```python
from build123d import *

# Parameters (mm, degrees)
F0_W       = 34
F0_H       = 18
F1_DEPTH   = 80
F2_SIZE2   = 7
F2_SIZE    = 17
F2_2_SIZE2 = 7
F2_2_SIZE  = 17
F3_T       = -1.2
F5_DEPTH   = 18.001
F6_R       = 1.2
F7_R       = 2.4


with BuildPart() as f1:
    # F0 (on Top) → F1 (new body)
    with BuildSketch(Plane.XY):
        Rectangle(F0_W, F0_H)
    extrude(amount=F1_DEPTH)

    # F2
    f2_edges = [f1.edges().sort_by_distance(p)[0] for p in [
        (-17, 0, 80),
    ]]
    f2_side = f1.faces().sort_by_distance((-17, 0, 40))[0]
    chamfer(f2_edges, length=F2_SIZE, length2=F2_SIZE2, reference=f2_side)

    # F2#2
    f2_2_edges = [f1.edges().sort_by_distance(p)[0] for p in [
        (17, 0, 80),
    ]]
    f2_2_side = f1.faces().sort_by_distance((17, 0, 40))[0]
    chamfer(f2_2_edges, length=F2_2_SIZE, length2=F2_2_SIZE2, reference=f2_2_side)

    # F3
    f3_openings = [f1.faces().sort_by_distance(p)[0] for p in [
        (0, 0, 80),
    ]]
    offset(amount=F3_T, openings=f3_openings)

    # F4 (on face) → F5 (cut, through all)
    with BuildSketch(Plane.XZ.offset(9)):
        Polygon((-6.7556277098, 80), (-14, 62.4065244382), (-14, 3), (14, 3), (14, 62.4065244382), (6.7556277098, 80), align=None)
    extrude(amount=-F5_DEPTH, mode=Mode.SUBTRACT)

    # F6
    f6_edges = [f1.edges().sort_by_distance(p)[0] for p in [
        (0, 7.8, 1.2),
        (-15.8, 7.8, 31.981305),
        (-15.8, -7.8, 31.981305),
        (15.8, -7.8, 31.981305),
        (15.8, 0, 1.2),
        (15.8, 7.8, 31.981305),
        (-15.8, 0, 1.2),
        (0, -7.8, 1.2),
        (-12.251126, -7.8, 71.381305),
        (12.251126, -7.8, 71.381305),
        (15.8, 0, 62.76261),
        (12.251126, 7.8, 71.381305),
        (-12.251126, 7.8, 71.381305),
        (-15.8, 0, 62.76261),
    ]]
    fillet(f6_edges, radius=F6_R)

    # F7
    f7_edges = [f1.edges().sort_by_distance(p)[0] for p in [
        (-17, 9, 31.5),
        (17, 9, 31.5),
        (-17, -9, 31.5),
        (-13.5, 9, 71.5),
        (-17, 0, 63),
        (-13.5, -9, 71.5),
        (13.5, -9, 71.5),
        (17, -9, 31.5),
        (13.5, 9, 71.5),
    ]]
    fillet(f7_edges, radius=F7_R)


solid = f1.part
```
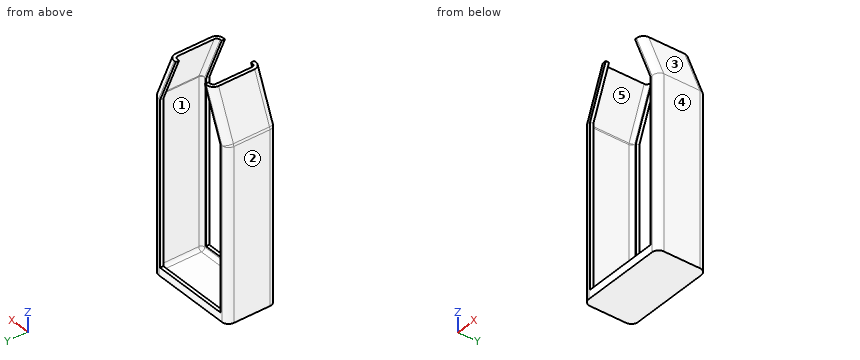
The listing builds one solid part. Answer for the finished solid, in the listing's coordinates (mm). Face numbers are marked on the shaded views. A direction names the side the tool comes from. Give positions to 0.01 mm unless a question says otherwise; leave off trailing zeros. Loops run counter-clockwise (first coordinate to the right, second up) from the corner with the lowest first, then second, coordinate; pieces in that order, holes last. Notation, with made-up numbers: (52, 19) - (59, 19) arc R8 ccw to (59, 33) - close; hole circle Ø2 at (-30, -22). An arc over 180 degrees is marked (long way). Return JSON: item names as keys, results as strings. Group by question number.
1. Find section A-A (z = 16). Write down the section's boundary in (x, y).
2. Which of the six approach directions +Z, -Z, +X, -X, +Y, -Y give full straight-line access (tool end or side, diameter ignored) to the marked faces 4 and 5?
3. Straight lines are drawn through the part: line 1 (X direction, y = 5.75, z = 32); line 2 (Z direction, x = -7, y = -3.5); line 3 (X direction, y = -5, z = 70). For each, find the intervals that lie inside material, in ascending order. Write a range as [from, to].
4. Determine the mould class of the marked faces 1, 2 and 3 for opening direction X: pulls with the +X half, pulls with the -X half, needs draft (parallel to the pull), parting line crosses it, or undercut.
5. Find section C-C (x = 5.5). Write down the section's boundary in (y, z), then the cut area to 3 significant figures.
6. Given pin 1 Ø0.6 at (y, z) = (-8.5, 44) entering from -X; pin 2 Ø1.3 at (y, z) = (8.5, 39.5) entering from +X; pin 3 Ø9 at (x, z) = (-6, 49.5) entering from +Y; pin 4 Ø4 at (x, y) = (-2.5, -1) entering from +Z, each flat-ended and moving along its own axis, determine where each tip first touches the part or whether it passes through.
7. Find section B-B (y = 3). Write down the section's boundary in (x, z).
Verdict:
{
 "1": {"outline": "(-17, -6.6) arc R2.4 ccw to (-14.6, -9) - (-14, -9) - (-14, -7.8) - (-14.6, -7.8) arc R1.2 cw to (-15.8, -6.6) - (-15.8, 6.6) arc R1.2 cw to (-14.6, 7.8) - (-14, 7.8) - (-14, 9) - (-14.6, 9) arc R2.4 ccw to (-17, 6.6) - close; (14, -9) - (14.6, -9) arc R2.4 ccw to (17, -6.6) - (17, 6.6) arc R2.4 ccw to (14.6, 9) - (14, 9) - (14, 7.8) - (14.6, 7.8) arc R1.2 cw to (15.8, 6.6) - (15.8, -6.6) arc R1.2 cw to (14.6, -7.8) - (14, -7.8) - close"},
 "2": {"face 4": "+Z, -Z, +X, +Y, -Y", "face 5": "none"},
 "3": {"line 1": "x = [-17, -15.8], [15.8, 17]", "line 2": "z = [0, 1.2]", "line 3": "x = [-14.12, -12.82], [12.82, 14.12]"},
 "4": {"face 1": "undercut", "face 2": "pulls with the -X half", "face 3": "pulls with the +X half"},
 "5": {"outline": "(-9, 0) - (9, 0) - (9, 3) - (7.8, 3) - (7.8, 2.4) arc R1.2 cw to (6.6, 1.2) - (-6.6, 1.2) arc R1.2 cw to (-7.8, 2.4) - (-7.8, 3) - (-9, 3) - close", "area": "26.5 mm^2"},
 "6": {"pin 1": "stops at x = -16.39", "pin 2": "stops at x = 16.65", "pin 3": "passes through", "pin 4": "stops at z = 1.2"},
 "7": {"outline": "(-17, 0) - (17, 0) - (17, 63) - (10, 80) - (8.7, 80) - (15.71, 62.98) arc R1.2 cw to (15.8, 62.53) - (15.8, 2.4) arc R1.2 cw to (14.6, 1.2) - (-14.6, 1.2) arc R1.2 cw to (-15.8, 2.4) - (-15.8, 62.53) arc R1.2 cw to (-15.71, 62.98) - (-8.7, 80) - (-10, 80) - (-16.82, 63.44) arc R2.4 ccw to (-17, 62.53) - close"}
}
